from build123d import *

# Parameters (mm, degrees)
BOSS_EXTRUDE1_DEPTH                   = 16.51
F_1_4_20_TAPPED_HOLE2_D               = 5.1054
F_1_4_20_TAPPED_HOLE2_DEPTH           = 16.51
F_1_4_20_TAPPED_HOLE2_TIP             = 1.533816902
F_1_4_20_TAPPED_HOLE2_ON_FACE_2_D     = 5.1054
F_1_4_20_TAPPED_HOLE2_ON_FACE_2_DEPTH = 16.51
F_1_4_20_TAPPED_HOLE2_ON_FACE_2_TIP   = 1.533816902
F_1_4_20_TAPPED_HOLE2_ON_FACE_3_D     = 5.1054
F_1_4_20_TAPPED_HOLE2_ON_FACE_3_DEPTH = 16.51
F_1_4_20_TAPPED_HOLE2_ON_FACE_3_TIP   = 1.533816902
F_1_4_20_TAPPED_HOLE2_ON_FACE_4_D     = 5.1054
F_1_4_20_TAPPED_HOLE2_ON_FACE_4_DEPTH = 16.51
F_1_4_20_TAPPED_HOLE2_ON_FACE_4_TIP   = 1.533816902
F_1_4_20_TAPPED_HOLE2_ON_FACE_5_D     = 5.1054
F_1_4_20_TAPPED_HOLE2_ON_FACE_5_DEPTH = 16.51
F_1_4_20_TAPPED_HOLE2_ON_FACE_5_TIP   = 1.533816902
F_1_4_20_TAPPED_HOLE2_ON_FACE_6_D     = 5.1054
F_1_4_20_TAPPED_HOLE2_ON_FACE_6_DEPTH = 16.51
F_1_4_20_TAPPED_HOLE2_ON_FACE_6_TIP   = 1.533816902
F_1_4_20_TAPPED_HOLE2_ON_FACE_7_D     = 5.1054
F_1_4_20_TAPPED_HOLE2_ON_FACE_7_DEPTH = 16.51
F_1_4_20_TAPPED_HOLE2_ON_FACE_7_TIP   = 1.533816902


with BuildPart() as part:
    # Sketch1 → Boss-Extrude1 (new, symmetric)
    with BuildSketch(Plane(origin=(0, 0, 0), x_dir=(1, 0, 0), z_dir=(0, 1, 0))):
        Polygon((-58.65878735, 0), (-29.329393675, -50.8), (29.329393675, -50.8), (58.65878735, 0), (29.329393675, 50.8), (-29.329393675, 50.8), align=None)
    extrude(amount=BOSS_EXTRUDE1_DEPTH, both=True)

    # 1/4-20 Tapped Hole2
    with Locations(Plane(origin=(-14.225163033, 16.51, -19.717380526), x_dir=(0, 0, 1), z_dir=(0, 1, 0))):
        with Locations((0, 0), (23.5570377, 22.079652882)):
            Hole(F_1_4_20_TAPPED_HOLE2_D / 2, depth=F_1_4_20_TAPPED_HOLE2_DEPTH)
            with Locations((0, 0, -(F_1_4_20_TAPPED_HOLE2_DEPTH + F_1_4_20_TAPPED_HOLE2_TIP / 2))):  # 118° drill point
                Cone(0, F_1_4_20_TAPPED_HOLE2_D / 2, F_1_4_20_TAPPED_HOLE2_TIP, mode=Mode.SUBTRACT)

    # 1/4-20 Tapped Hole2 on face 2
    with Locations(Plane(origin=(41.36951867, 0.562395416, -29.945891779), x_dir=(0.500000174844, 0, 0.866025302838), z_dir=(0.866025302838, 0, -0.500000174844))):
        with Locations((0, 0)):
            Hole(F_1_4_20_TAPPED_HOLE2_ON_FACE_2_D / 2, depth=F_1_4_20_TAPPED_HOLE2_ON_FACE_2_DEPTH)
            with Locations((0, 0, -(F_1_4_20_TAPPED_HOLE2_ON_FACE_2_DEPTH + F_1_4_20_TAPPED_HOLE2_ON_FACE_2_TIP / 2))):  # 118° drill point
                Cone(0, F_1_4_20_TAPPED_HOLE2_ON_FACE_2_D / 2, F_1_4_20_TAPPED_HOLE2_ON_FACE_2_TIP, mode=Mode.SUBTRACT)

    # 1/4-20 Tapped Hole2 on face 3
    with Locations(Plane(origin=(43.994090512, 0, 25.4), x_dir=(-0.500000174844, 0, 0.866025302838), z_dir=(0.866025302838, 0, 0.500000174844))):
        with Locations((0, 0)):
            Hole(F_1_4_20_TAPPED_HOLE2_ON_FACE_3_D / 2, depth=F_1_4_20_TAPPED_HOLE2_ON_FACE_3_DEPTH)
            with Locations((0, 0, -(F_1_4_20_TAPPED_HOLE2_ON_FACE_3_DEPTH + F_1_4_20_TAPPED_HOLE2_ON_FACE_3_TIP / 2))):  # 118° drill point
                Cone(0, F_1_4_20_TAPPED_HOLE2_ON_FACE_3_D / 2, F_1_4_20_TAPPED_HOLE2_ON_FACE_3_TIP, mode=Mode.SUBTRACT)

    # 1/4-20 Tapped Hole2 on face 4
    with Locations(Plane(origin=(-0.767217268, 0.17198146, 50.8), x_dir=(1, 0, 0), z_dir=(0, 0, 1))):
        with Locations((0, 0)):
            Hole(F_1_4_20_TAPPED_HOLE2_ON_FACE_4_D / 2, depth=F_1_4_20_TAPPED_HOLE2_ON_FACE_4_DEPTH)
            with Locations((0, 0, -(F_1_4_20_TAPPED_HOLE2_ON_FACE_4_DEPTH + F_1_4_20_TAPPED_HOLE2_ON_FACE_4_TIP / 2))):  # 118° drill point
                Cone(0, F_1_4_20_TAPPED_HOLE2_ON_FACE_4_D / 2, F_1_4_20_TAPPED_HOLE2_ON_FACE_4_TIP, mode=Mode.SUBTRACT)

    # 1/4-20 Tapped Hole2 on face 5
    with Locations(Plane(origin=(-38.190702716, -1.730660851, 35.451762519), x_dir=(-0.500000174844, 0, -0.866025302838), z_dir=(-0.866025302838, 0, 0.500000174844))):
        with Locations((0, 0)):
            Hole(F_1_4_20_TAPPED_HOLE2_ON_FACE_5_D / 2, depth=F_1_4_20_TAPPED_HOLE2_ON_FACE_5_DEPTH)
            with Locations((0, 0, -(F_1_4_20_TAPPED_HOLE2_ON_FACE_5_DEPTH + F_1_4_20_TAPPED_HOLE2_ON_FACE_5_TIP / 2))):  # 118° drill point
                Cone(0, F_1_4_20_TAPPED_HOLE2_ON_FACE_5_D / 2, F_1_4_20_TAPPED_HOLE2_ON_FACE_5_TIP, mode=Mode.SUBTRACT)

    # 1/4-20 Tapped Hole2 on face 6
    with Locations(Plane(origin=(-48.031402305, -4.745159271, -18.407170849), x_dir=(0.500000174844, 0, -0.866025302838), z_dir=(-0.866025302838, 0, -0.500000174844))):
        with Locations((0, 0)):
            Hole(F_1_4_20_TAPPED_HOLE2_ON_FACE_6_D / 2, depth=F_1_4_20_TAPPED_HOLE2_ON_FACE_6_DEPTH)
            with Locations((0, 0, -(F_1_4_20_TAPPED_HOLE2_ON_FACE_6_DEPTH + F_1_4_20_TAPPED_HOLE2_ON_FACE_6_TIP / 2))):  # 118° drill point
                Cone(0, F_1_4_20_TAPPED_HOLE2_ON_FACE_6_D / 2, F_1_4_20_TAPPED_HOLE2_ON_FACE_6_TIP, mode=Mode.SUBTRACT)

    # 1/4-20 Tapped Hole2 on face 7
    with Locations(Plane(origin=(3.490061769, -2.916627308, -50.8), x_dir=(-1, 0, 0), z_dir=(0, 0, -1))):
        with Locations((0, 0)):
            Hole(F_1_4_20_TAPPED_HOLE2_ON_FACE_7_D / 2, depth=F_1_4_20_TAPPED_HOLE2_ON_FACE_7_DEPTH)
            with Locations((0, 0, -(F_1_4_20_TAPPED_HOLE2_ON_FACE_7_DEPTH + F_1_4_20_TAPPED_HOLE2_ON_FACE_7_TIP / 2))):  # 118° drill point
                Cone(0, F_1_4_20_TAPPED_HOLE2_ON_FACE_7_D / 2, F_1_4_20_TAPPED_HOLE2_ON_FACE_7_TIP, mode=Mode.SUBTRACT)


solid = part.part
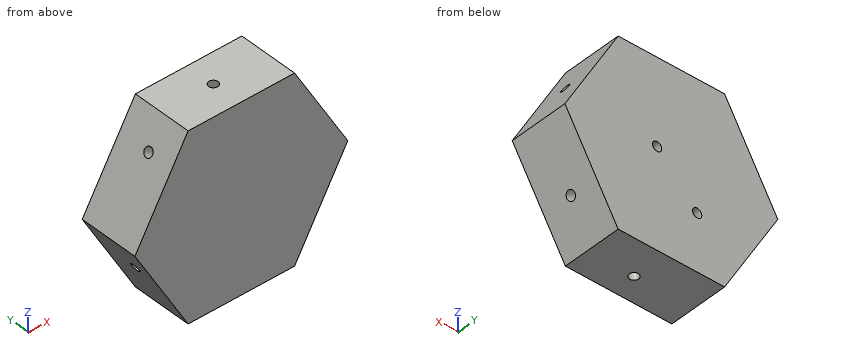
Geometry: final body of the model. Coordinates: model frame, mm. Round coordinates to 2 decimals unless told otherwise and drop trailing zeros. Loops run counter-clockwise (first coordinate to the right, second up) from the corner with the lowest first, then second, coordinate; pieces in that order, holes last.
Q1. Material intervals for L1, parallel to X at y = 13.5, z = -17.5; L2, parallel to Z at x = -14, y = 7; L3, parallel to Z at x = -31.5, y = -2.5, sorted ascending.
Q2. Section B-B on y = 8.5. Return loops of the section in (x, z), plus the area to 3 significant figures.
Q3. Pin query (flat end, axial travel): P1, Ø4, axis at y = 9.5, z = 1, coming from the +X side; P2, Ø5, axis at x = -43, z = 34.5, coming from the -Y side; P3, Ø3, axis at x = 3.49, y = -2.92, coming from the -Z side; P4, Ø3, axis at x = 7.85, z = 3.84, coming from the +Y side. Return the tip coordinate at first contact, or that it passes through.
Q4. Section C-C on x = -51. Return loops of the section in (y, z).
Q5. Section D-D on z = -5. Return loops of the section in (x, y), plus the area to 3 significant figures.
Q6. Section A-A on y = -10. Return loops of the section in (x, z), plus the area to 3 significant figures.
Evaluation:
1. L1: x = -48.56 to -15.49, -12.96 to 48.56
1. L2: z = -50.8 to -22.26, -17.17 to 50.8
1. L3: z = -47.04 to 28.78, 34.4 to 47.04
2. outline: (-58.66, 0) - (-29.33, -50.8) - (29.33, -50.8) - (58.66, 0) - (29.33, 50.8) - (-29.33, 50.8) - close; hole circle Ø5.11 at (-14.23, -19.72); hole circle Ø5.11 at (7.85, 3.84)
2. area: 8,900 mm2
3. P1: stops at x = 58.66
3. P2: passes through
3. P3: stops at z = -33.66
3. P4: stops at y = -0.63
4. outline: (-16.51, -13.27) - (16.51, -13.27) - (16.51, 13.27) - (-16.51, 13.27) - close
5. outline: (-55.77, -16.51) - (55.77, -16.51) - (55.77, 16.51) - (-55.77, 16.51) - close
5. area: 3,680 mm2
6. outline: (-58.66, 0) - (-29.33, -50.8) - (29.33, -50.8) - (58.66, 0) - (29.33, 50.8) - (-29.33, 50.8) - close
6. area: 8,940 mm2
